Design review of the part built by this model. Coordinates are the model's own, in mm. Give positions to 0.01 mm unless a question says otherwise; leave off trailing zeros. Write each loop counter-clockwise with the first axis right and the second up, starting at its lowest first coordinate (ties: lowest second). Pieces come first, ordered by that corner, then holes.
```python
from build123d import *

# Parameters (mm, degrees)
SKETCH1_R           = 1.5
SKETCH1_W           = 13
SKETCH1_H           = 17.5
BOSS_EXTRUDE1_DEPTH = 3


with BuildPart() as part:
    # Sketch1 → Boss-Extrude1 (new body)
    with BuildSketch(Plane.XY):
        with BuildLine():
            Line((75, 50), (-75, 50))
            ThreePointArc((-75, 50), (-82.071067812, 47.071067812), (-85, 40))
            Line((-85, 40), (-85, -40))
            ThreePointArc((-85, -40), (-82.071067812, -47.071067812), (-75, -50))
            Line((-75, -50), (75, -50))
            ThreePointArc((75, -50), (82.071067812, -47.071067812), (85, -40))
            Line((85, -40), (85, 40))
            ThreePointArc((85, 40), (82.071067812, 47.071067812), (75, 50))
        make_face()
        with Locations((-75, -40)):
            Circle(SKETCH1_R, mode=Mode.SUBTRACT)
        with BuildLine():
            ThreePointArc((-72.18, -19.8), (-73.68, -18.3), (-72.18, -16.8))
            Line((-72.18, -16.8), (-70.608485706, -16.8))
            ThreePointArc((-70.608485706, -16.8), (-70.18, -16.74), (-69.751514294, -16.8))
            Line((-69.751514294, -16.8), (-68.18, -16.8))
            ThreePointArc((-68.18, -16.8), (-66.68, -18.3), (-68.18, -19.8))
            Line((-68.18, -19.8), (-69.751514294, -19.8))
            ThreePointArc((-69.751514294, -19.8), (-70.18, -19.86), (-70.608485706, -19.8))
            Line((-70.608485706, -19.8), (-72.18, -19.8))
        make_face(mode=Mode.SUBTRACT)
        with BuildLine():
            Line((25, -46.257829906), (-25, -46.257829906))
            ThreePointArc((-25, -46.257829906), (-30, -41.257829906), (-25, -36.257829906))
            Line((-25, -36.257829906), (25, -36.257829906))
            ThreePointArc((25, -36.257829906), (30, -41.257829906), (25, -46.257829906))
        make_face(mode=Mode.SUBTRACT)
        with Locations((75, -40)):
            Circle(SKETCH1_R, mode=Mode.SUBTRACT)
        with BuildLine():
            ThreePointArc((10.37, -19.8), (8.87, -18.3), (10.37, -16.8))
            Line((10.37, -16.8), (11.941514294, -16.8))
            ThreePointArc((11.941514294, -16.8), (12.37, -16.74), (12.798485706, -16.8))
            Line((12.798485706, -16.8), (14.37, -16.8))
            ThreePointArc((14.37, -16.8), (15.87, -18.3), (14.37, -19.8))
            Line((14.37, -19.8), (12.798485706, -19.8))
            ThreePointArc((12.798485706, -19.8), (12.37, -19.86), (11.941514294, -19.8))
            Line((11.941514294, -19.8), (10.37, -19.8))
        make_face(mode=Mode.SUBTRACT)
        with BuildLine():
            Line((28.5, -7.351514294), (28.5, -5.28))
            ThreePointArc((28.5, -5.28), (30, -3.78), (31.5, -5.28))
            Line((31.5, -5.28), (31.5, -7.351514294))
            ThreePointArc((31.5, -7.351514294), (31.544927183, -7.563666923), (31.56, -7.78))
            ThreePointArc((31.56, -7.78), (31.544927183, -7.996333077), (31.5, -8.208485706))
            Line((31.5, -8.208485706), (31.5, -10.28))
            ThreePointArc((31.5, -10.28), (30, -11.78), (28.5, -10.28))
            Line((28.5, -10.28), (28.5, -8.208485706))
            ThreePointArc((28.5, -8.208485706), (28.44, -7.78), (28.5, -7.351514294))
        make_face(mode=Mode.SUBTRACT)
        with BuildLine():
            ThreePointArc((63.5, -1.95), (65, -0.45), (66.5, -1.95))
            Line((66.5, -1.95), (66.5, -18.05))
            ThreePointArc((66.5, -18.05), (65, -19.55), (63.5, -18.05))
            Line((63.5, -18.05), (63.5, -1.95))
        make_face(mode=Mode.SUBTRACT)
        with BuildLine():
            ThreePointArc((-67.18, 31.5), (-65.68, 30), (-67.18, 28.5))
            Line((-67.18, 28.5), (-68.751514294, 28.5))
            ThreePointArc((-68.751514294, 28.5), (-69.18, 28.44), (-69.608485706, 28.5))
            Line((-69.608485706, 28.5), (-71.18, 28.5))
            ThreePointArc((-71.18, 28.5), (-72.68, 30), (-71.18, 31.5))
            Line((-71.18, 31.5), (-69.608485706, 31.5))
            ThreePointArc((-69.608485706, 31.5), (-69.18, 31.56), (-68.751514294, 31.5))
            Line((-68.751514294, 31.5), (-67.18, 31.5))
        make_face(mode=Mode.SUBTRACT)
        with Locations((-75, 40)):
            Circle(SKETCH1_R, mode=Mode.SUBTRACT)
        with BuildLine():
            ThreePointArc((31.5, 5.28), (30, 3.78), (28.5, 5.28))
            Line((28.5, 5.28), (28.5, 7.351514294))
            ThreePointArc((28.5, 7.351514294), (28.44, 7.78), (28.5, 8.208485706))
            Line((28.5, 8.208485706), (28.5, 10.28))
            ThreePointArc((28.5, 10.28), (30, 11.78), (31.5, 10.28))
            Line((31.5, 10.28), (31.5, 8.208485706))
            ThreePointArc((31.5, 8.208485706), (31.544927183, 7.996333077), (31.56, 7.78))
            ThreePointArc((31.56, 7.78), (31.544927183, 7.563666923), (31.5, 7.351514294))
            Line((31.5, 7.351514294), (31.5, 5.28))
        make_face(mode=Mode.SUBTRACT)
        with Locations((65, 20)):
            Rectangle(SKETCH1_W, SKETCH1_H, mode=Mode.SUBTRACT)
        with BuildLine():
            ThreePointArc((3.75, 28.5), (2.25, 30), (3.75, 31.5))
            Line((3.75, 31.5), (5.321514294, 31.5))
            ThreePointArc((5.321514294, 31.5), (5.75, 31.56), (6.178485706, 31.5))
            Line((6.178485706, 31.5), (7.75, 31.5))
            ThreePointArc((7.75, 31.5), (9.25, 30), (7.75, 28.5))
            Line((7.75, 28.5), (6.178485706, 28.5))
            ThreePointArc((6.178485706, 28.5), (5.75, 28.44), (5.321514294, 28.5))
            Line((5.321514294, 28.5), (3.75, 28.5))
        make_face(mode=Mode.SUBTRACT)
        with BuildLine():
            ThreePointArc((-25, 36.257829906), (-30, 41.257829906), (-25, 46.257829906))
            Line((-25, 46.257829906), (25, 46.257829906))
            ThreePointArc((25, 46.257829906), (30, 41.257829906), (25, 36.257829906))
            Line((25, 36.257829906), (-25, 36.257829906))
        make_face(mode=Mode.SUBTRACT)
        with Locations((75, 40)):
            Circle(SKETCH1_R, mode=Mode.SUBTRACT)
    extrude(amount=BOSS_EXTRUDE1_DEPTH)


solid = part.part
```
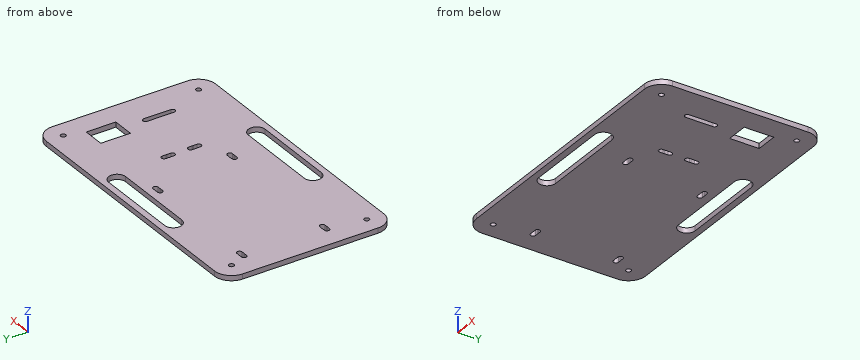
(1) To check wall thickness, follow L1, parallel to Y at x = -68.5, z = 2.1; L2, parallel to X at y = -10, z = 0.65; L3, parallel to Y at x = 75, z = 2.2. State the ranges of each line that lie inside material, in increasing order.
Resolved:
L1: y = -50 to -19.8, -16.8 to 28.5, 31.5 to 50
L2: x = -85 to 28.5, 31.5 to 63.5, 66.5 to 85
L3: y = -50 to -41.5, -38.5 to 38.5, 41.5 to 50
(2) Consider section B-B, the plane z = 1.5. Give the number of separate pieces and of enclosed holes in the cut face, then the cut area to 3 significant figures.
Resolved:
separate pieces: 1
enclosed holes: 14
area: 15,300 mm2
(3) Clearance check with a flat-ended pin moving along its axis: P1, Ø6, axis at x = -62, y = -30, coming from the -Z side. State where the tip first meets the part, or that it passes through.
Resolved:
P1: stops at z = 0
(4) Consider section A-A, the plane x = -22. Give the boundary of the cut face in (y, z), then the cut area to 3 significant figures.
Resolved:
outline: (-50, 0) - (-46.26, 0) - (-46.26, 3) - (-50, 3) - close; (-36.26, 0) - (36.26, 0) - (36.26, 3) - (-36.26, 3) - close; (46.26, 0) - (50, 0) - (50, 3) - (46.26, 3) - close
area: 240 mm2
